Geometry check sheet. Reference: the model listing, model coordinates, mm. A direction names the side the tool comes from. Round coordinates to 2 decimals unless told otherwise and drop trailing zeros. Order: outer loops, then holes, each group sorted by start corner. A loop starts at its lowest first (then second) coordinate and runs counter-clockwise, first axis right, second up.
(1) Sectioned sample at A-A (y = 12). Record the boundary of the cut face in (x, z).
(2) Sectioned sample at D-D (x = 0). Record the boundary of the cut face in (y, z).
(3) Material ranges on line 1 along X through (y, z) = (1, 6.25); line 2 along X through (y, z) = (28.5, 4.25); line 3 along Y through (x, z) = (-20, 3), recorded low to high.
(4) Sectioned sample at C-C (y = 32). Record the boundary of the cut face in (x, z), plus the area to 3 significant figures.
(5) Go/stop test with a flat-tipped pin: pin 1 (5 mm diameter, centred on x = 13.5, z = 6, fed in from -Y). Record where the tip stops, or that it passes through.
(6) Sectioned sample at B-B (z = 2). Record the boundary of the cut face in (x, y), plus the area to 3 significant figures.
(7) Set-up check for faces 1 (the face through (-3, 37, 0)), 2 (the face through (18.5, 7, 5)): record each of +Z, -Z, +X, -X, +Y, -Y from which the full face is reachable in a straight line by a thin tool's end or side.
(8) Release check for a two-part mould opening along X. For faces 3 (the face through (20, -5, 5)), 4 (the face through (-22.5, 7, 5)), 5 (the face through (-18.5, 7, 5)), 6 (the face through (0, 37, 5)) record: +X half, -X half, draft (parallel to the pull), parting line (faces both ways), or undercut.
from build123d import *

# Parameters (mm, degrees)
BOSS_EXTRUDE1_DEPTH = 10
SKETCH2_W           = 4
SKETCH2_H           = 10
BOSS_EXTRUDE2_DEPTH = 5


with BuildPart() as part:
    # Sketch1 → Boss-Extrude1 (new body)
    with BuildSketch(Plane.XY):
        with BuildLine():
            Line((18.5, 18.5), (18.5, 0))
            Line((18.5, 0), (22.5, 0))
            Line((22.5, 0), (22.5, 18.5))
            ThreePointArc((22.5, 18.5), (0, 41), (-22.5, 18.5))
            Line((-22.5, 18.5), (-22.5, 0))
            Line((-22.5, 0), (-18.5, 0))
            Line((-18.5, 0), (-18.5, 18.5))
            ThreePointArc((-18.5, 18.5), (0, 37), (18.5, 18.5))
        make_face()
    extrude(amount=BOSS_EXTRUDE1_DEPTH)

    # Sketch2 → Boss-Extrude2 (add)
    with BuildSketch(Plane.XZ):
        with Locations((20.5, 5)):
            Rectangle(SKETCH2_W, SKETCH2_H)
        with Locations((-20.5, 5)):
            Rectangle(SKETCH2_W, SKETCH2_H)
    extrude(amount=BOSS_EXTRUDE2_DEPTH)


solid = part.part
Answer below:
1. outline: (-22.5, 0) - (-18.5, 0) - (-18.5, 10) - (-22.5, 10) - close; (18.5, 0) - (22.5, 0) - (22.5, 10) - (18.5, 10) - close
2. outline: (37, 0) - (41, 0) - (41, 10) - (37, 10) - close
3. line 1: x = -22.5 to -18.5, 18.5 to 22.5
3. line 2: x = -20.16 to -15.56, 15.56 to 20.16
3. line 3: y = -5 to 28.81
4. outline: (-18, 0) - (-12.65, 0) - (-12.65, 10) - (-18, 10) - close; (12.65, 0) - (18, 0) - (18, 10) - (12.65, 10) - close
4. area: 107 mm2
5. pin 1: stops at y = 27.79
6. outline: (-22.5, -5) - (-18.5, -5) - (-18.5, 18.5) arc R18.5 cw to (18.5, 18.5) - (18.5, -5) - (22.5, -5) - (22.5, 18.5) arc R22.5 ccw to (-22.5, 18.5) - close
6. area: 446 mm2
7. face 1: -Z, +X, -X, +Y, -Y
7. face 2: +Z, -Z, -Y
8. face 3: draft
8. face 4: -X half
8. face 5: undercut
8. face 6: undercut
